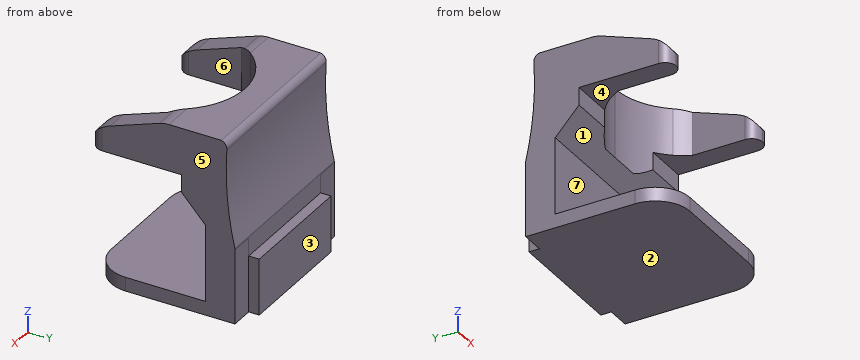
from build123d import *

# Parameters (mm, degrees)
BOSS_EXTRUDE2_DEPTH = 17.8
CUT_EXTRUDE1_DEPTH  = 15.6
CUT_EXTRUDE2_DEPTH  = 15.6


with BuildPart() as part:
    # Sketch2 → Boss-Extrude2 (new, symmetric)
    with BuildSketch(Plane(origin=(0, 0, 0), x_dir=(0, 0, -1), z_dir=(1, 0, 0))):
        with BuildLine():
            Line((0, 15.50389008), (-11.8, 15.50389008))
            Line((-11.8, 15.50389008), (-11.8, 13.30389008))
            Line((-11.8, 13.30389008), (-15.8, 13.30389008))
            ThreePointArc((-15.8, 13.30389008), (-15.869442202, 13.299917081), (-15.937978141, 13.288049932))
            ThreePointArc((-15.937978141, 13.288049932), (-26.064403897, 11.700216575), (-36.314108018, 11.60389008))
            ThreePointArc((-36.314108018, 11.60389008), (-37.313669561, 11.31470673), (-37.9, 10.455074886))
            Line((-37.9, 10.455074886), (-37.9, -0.544925114))
            ThreePointArc((-37.9, -0.544925114), (-37.813111141, -1.55413735), (-37.555001853, -2.533646721))
            Line((-37.555001853, -2.533646721), (-33.85, -12.890912831))
            ThreePointArc((-33.85, -12.890912831), (-32.58061565, -15.162493454), (-30.64, -16.89610992))
            Line((-30.64, -16.89610992), (-28.1, -16.89610992))
            Line((-28.1, -16.89610992), (-28.1, 2.10389008))
            Line((-28.1, 2.10389008), (-24.4, 2.10389008))
            Line((-24.4, 2.10389008), (-19, 7.10389008))
            Line((-19, 7.10389008), (-2.9, 7.10389008))
            Line((-2.9, 7.10389008), (-2.9, -16.89610992))
            Line((-2.9, -16.89610992), (0, -16.89610992))
            Line((0, -16.89610992), (0, 15.50389008))
        make_face()
    extrude(amount=BOSS_EXTRUDE2_DEPTH, both=True)

    # Sketch3 → Cut-Extrude1 (cut)
    with BuildSketch(Plane.XY.offset(37.9)):
        with BuildLine():
            Line((-13.2, -14.59610992), (-13.2, -16.89610992))
            Line((-13.2, -16.89610992), (13.2, -16.89610992))
            Line((13.2, -16.89610992), (13.2, -14.59610992))
            Line((13.2, -14.59610992), (13.2, -3.49610992))
            ThreePointArc((13.2, -3.49610992), (12.380923678, -1.966255492), (11.385353215, -0.544925114))
            Line((11.385353215, -0.544925114), (-11.385353215, -0.544925114))
            ThreePointArc((-11.385353215, -0.544925114), (-12.380923678, -1.966255492), (-13.2, -3.49610992))
            Line((-13.2, -3.49610992), (-13.2, -14.59610992))
        make_face()
        with BuildLine():
            ThreePointArc((0, 4.955074886), (-6.322109375, 3.508041139), (-11.385353215, -0.544925114))
            Line((-11.385353215, -0.544925114), (11.385353215, -0.544925114))
            ThreePointArc((11.385353215, -0.544925114), (6.322109375, 3.508041139), (0, 4.955074886))
        make_face()
        with BuildLine():
            Line((-15.5, -16.89610992), (-13.2, -16.89610992))
            Line((-13.2, -16.89610992), (-13.2, -14.59610992))
            ThreePointArc((-13.2, -14.59610992), (-13.873654403, -16.222455516), (-15.5, -16.89610992))
        make_face()
        with BuildLine():
            Line((-17.8, -16.89610992), (-15.5, -16.89610992))
            ThreePointArc((-15.5, -16.89610992), (-17.126345597, -16.222455516), (-17.8, -14.59610992))
            Line((-17.8, -14.59610992), (-17.8, -16.89610992))
        make_face()
        with BuildLine():
            Line((13.2, -14.59610992), (13.2, -16.89610992))
            Line((13.2, -16.89610992), (15.5, -16.89610992))
            ThreePointArc((15.5, -16.89610992), (13.873654403, -16.222455516), (13.2, -14.59610992))
        make_face()
        with BuildLine():
            ThreePointArc((17.8, -14.59610992), (17.126345597, -16.222455516), (15.5, -16.89610992))
            Line((15.5, -16.89610992), (17.8, -16.89610992))
            Line((17.8, -16.89610992), (17.8, -14.59610992))
        make_face()
    extrude(amount=-CUT_EXTRUDE1_DEPTH, mode=Mode.SUBTRACT)

    # Sketch4 → Cut-Extrude2 (cut)
    with BuildSketch(Plane.XY):
        Polygon((-12.875, 15.50389008), (-12.875, 13.30389008), (-17.8, 13.288049932), (-17.8, 15.50389008), align=None)
        Polygon((12.875, 15.50389008), (17.8, 15.50389008), (17.8, 13.288049932), (12.875, 13.30389008), align=None)
        with BuildLine():
            Line((17.8, -9.604528344), (17.8, -16.89610992))
            Line((17.8, -16.89610992), (10.508418424, -16.89610992))
            ThreePointArc((10.508418424, -16.89610992), (15.664345202, -14.760455122), (17.8, -9.604528344))
        make_face()
        with BuildLine():
            Line((-17.8, -9.604528344), (-17.8, -16.89610992))
            Line((-17.8, -16.89610992), (-10.508418424, -16.89610992))
            ThreePointArc((-10.508418424, -16.89610992), (-15.664345202, -14.760455122), (-17.8, -9.604528344))
        make_face()
    extrude(amount=CUT_EXTRUDE2_DEPTH, mode=Mode.SUBTRACT)


solid = part.part
Read the model definition and answer for the solid it produces. Units are mm, in the model's axes. Face numbers are marked on the shaded views. A direction names the side the tool comes from. Give positions to 0.01 mm unless a question says otherwise; leave off trailing zeros. Write each loop counter-clockwise with the first axis right and the second up, starting at its lowest first coordinate (ties: lowest second). Pieces come first, ordered by that corner, then holes. Notation, with made-up numbers: (39.25, 26.25) - (64.25, 26.25) arc R28 ccw to (64.25, 49.25) - close; hole circle Ø6 at (59.5, 85). An arc over 180 degrees is marked (long way). Use CSV: the item, a comma, the result in double quotes. Start each with the question number.
Item 1: For the marked faces 5, 6 and 7, determine the directions among +Z, -Z, +X, -X, +Y, -Y from which every point of the face is accessible in a straight line to the end or side of a thin tool.
Item 2: The part is cut by section D-D, the plane x = -4.5. Give the vertices of the cut face in (y, z).
Item 3: Flat-ended cylindrical pins translate along their axes: P1, Ø8, axis at x = 12, y = -8, coming from the +Z side; P2, Ø0.7, axis at y = 15, z = 3.5, coming from the -X side (3 decimals); P3, Ø7, axis at x = 0.5, y = -9.5, coming from the +Z side. Find the tip coordinate at first contact, or state that the pin passes through.
Item 4: The part is cut by section B-B, the plane z = 13. Give the vertices of the cut face in (x, y) (3 decimals), and give its area (3 significant figures).
Item 5: The part is cut by section A-A, the plane y = 6. Give the vertices of the cut face in (x, z).
Item 6: The part is cut by section C-C, the plane y = -6. Give the vertices of the cut face in (x, z).
Item 7: The mould has two halves that part along Z. Classify the marked faces 1, 2, 3 and 4: pulls with the +Z half, pulls with the -Z half, needs draft (parallel to the pull), parting line crosses it, or undercut.
Item 8: Consider line 1 (Y direction, x = 11, z = 9); line 2 (Z direction, x = -4, y = -13.5); line 3 (Y direction, x = -10, z = 25). Determine where each line is inside the solid, lowest interval first.
Taken from the geometry:
1,face 5,"+Z, -Z, +X, +Y, -Y"
1,face 6,"+Z, -Y"
1,face 7,"+X, -X, -Y"
2,outline,"(-16.9, 0) - (15.5, 0) - (15.5, 11.8) - (13.3, 11.8) - (13.3, 15.8) arc R0.61 ccw to (13.29, 15.94) arc R70.2 cw to (11.6, 36.31) arc R1.54 ccw to (10.46, 37.9) - (4.24, 37.9) - (4.24, 22.3) - (4.05, 22.3) - (7.1, 19) - (7.1, 2.9) - (-16.9, 2.9) - close"
3,P1,"z = 36.96"
3,P2,"x = -12.875"
3,P3,"z = 2.9"
4,outline,"(-17.8, 7.104) - (17.8, 7.104) - (17.8, 13.288) - (12.875, 13.304) - (-12.875, 13.304) - (-17.8, 13.288) - close"
4,area,"221 mm2"
5,outline,"(-17.8, 0) - (17.8, 0) - (17.8, 2.9) - (-17.8, 2.9) - close; (-17.8, 20.19) - (17.8, 20.19) - (17.8, 37.9) - (-17.8, 37.9) - close"
6,outline,"(-17.8, 0) - (17.8, 0) - (17.8, 2.9) - (-17.8, 2.9) - close; (-17.8, 28.1) - (-13.2, 28.1) - (-13.2, 36.32) - (-17.8, 36.32) - close; (13.2, 28.1) - (17.8, 28.1) - (17.8, 36.32) - (13.2, 36.32) - close"
7,face 1,"undercut"
7,face 2,"pulls with the -Z half"
7,face 3,"needs draft"
7,face 4,"undercut"
8,line 1,"7.1 to 15.5"
8,line 2,"0 to 2.9"
8,line 3,"2.1 to 11.8"
